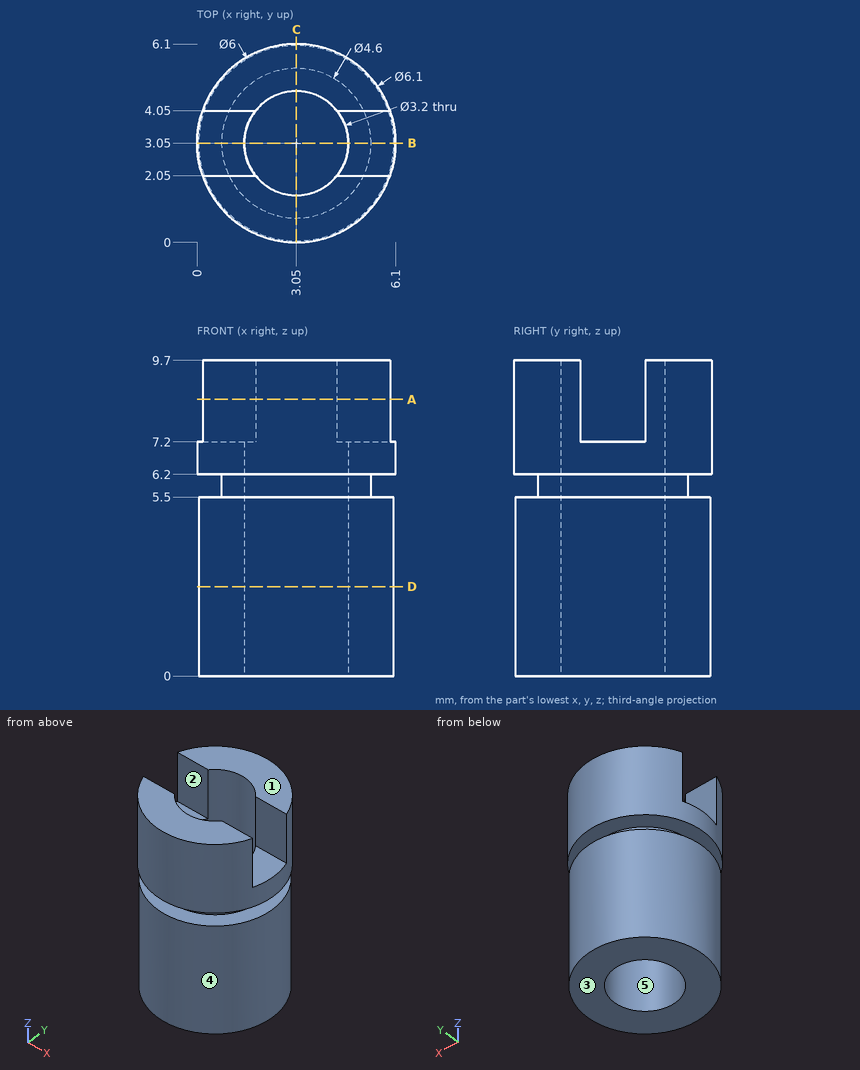
The figure shows three views and two pictorial views of one solid part (mm, origin at its lowest corner). Answer the questions. A direction names the side the tool comes from. Coordinates: 2 decimals unless noted, no trailing zeros. Write each loop counter-clockwise with the first axis right and the second up, starting at its lowest first coordinate (ties: lowest second). Pieces come first, ordered by that corner, then holes.
1. For the marked faces 1 and 2, determine the directions among +Z, -Z, +X, -X, +Y, -Y from which every point of the face is accessible in a straight line to the end or side of a thin tool.
Results list:
face 1: +Z, +X, -X, +Y, -Y
face 2: +Z, +X, -X
2. Consider line 1 along Z through (x, y) = (1.75, 5); line 2 along X through (y, z) = (3, 2.25); line 3 along Y through (x, z) = (3.05, 6.5). Determine where each line is inside the solid, lowest interval first.
Results list:
line 1: z = 0 to 5.5, 6.2 to 9.7
line 2: x = 0.05 to 1.45, 4.65 to 6.05
line 3: y = 0 to 1.45, 4.65 to 6.1
3. The part is cut by section D-D, the plane z = 2.75. Write down the section's boundary in (x, y).
Results list:
outline: circle Ø6 at (3.05, 3.05); hole circle Ø3.2 at (3.05, 3.05)
4. Flat-ended cylindrical pins translate along their axes: pin 1 (2 mm diameter, centred on x = 5, z = 8.5, fed in from +Y); pin 2 (3 mm diameter, centred on x = 1.5, z = 8, fed in from -Y); pin 3 (0.5 mm diameter, centred on x = 5.5, y = 3, fed in from +Z); pin 4 (0.8 mm diameter, centred on x = 1.5, z = 8, fed in from -Y). Find the tip coordinate at first contact, or state that the pin passes through.
Results list:
pin 1: stops at y = 5.95
pin 2: stops at y = 0
pin 3: stops at z = 7.2
pin 4: stops at y = 0.23
5. The part is cut by section A-A, the plane z = 8.5. Write down the section's boundary in (x, y).
Results list:
outline: (0.17, 2.05) arc R3.05 ccw to (5.93, 2.05) - (4.3, 2.05) arc R1.6 cw to (1.8, 2.05) - close; (0.17, 4.05) - (1.8, 4.05) arc R1.6 cw to (4.3, 4.05) - (5.93, 4.05) arc R3.05 ccw to start
6. The part is cut by section C-C, the plane x = 3.05. Write down the section's boundary in (y, z).
Results list:
outline: (0, 6.2) - (0.75, 6.2) - (0.75, 5.5) - (0.05, 5.5) - (0.05, 0) - (1.45, 0) - (1.45, 9.7) - (0, 9.7) - close; (4.65, 0) - (6.05, 0) - (6.05, 5.5) - (5.35, 5.5) - (5.35, 6.2) - (6.1, 6.2) - (6.1, 9.7) - (4.65, 9.7) - close
7. The part is cut by section B-B, the plane y = 3.05. Write down the section's boundary in (x, z), and give its area (3 significant figures).
Results list:
outline: (0, 6.2) - (0.75, 6.2) - (0.75, 5.5) - (0.05, 5.5) - (0.05, 0) - (1.45, 0) - (1.45, 7.2) - (0, 7.2) - close; (4.65, 0) - (6.05, 0) - (6.05, 5.5) - (5.35, 5.5) - (5.35, 6.2) - (6.1, 6.2) - (6.1, 7.2) - (4.65, 7.2) - close
area: 19.3 mm2
8. For a pull along X with two mould halves and no side action, classify the marked faces 3, 4 and 5 as +X half, -X half, draft (parallel to the pull), parting line (faces both ways), or undercut.
Results list:
face 3: draft
face 4: parting line
face 5: undercut
